```python
from build123d import *

# Parameters (mm, degrees)
ESQUISSE1_R        = 1.5
BOSS_EXTRU_1_DEPTH = 5


with BuildPart() as part:
    # Esquisse1 → Boss.-Extru.1 (new body)
    with BuildSketch(Plane(origin=(0, 0, 0), x_dir=(0, -1, 0), z_dir=(-1, 0, 0))):
        with BuildLine():
            Line((-5, 5), (-5, 0))
            Line((-5, 0), (0, 0))
            Line((0, 0), (0, 5))
            ThreePointArc((0, 5), (-2.5, 7.5), (-5, 5))
        make_face()
        with Locations(Location((-2.5, 5, 0), (0, 0, 270))):  # turned: the seam where the file's is
            Circle(ESQUISSE1_R, mode=Mode.SUBTRACT)
    extrude(amount=-BOSS_EXTRU_1_DEPTH)


solid = part.part
```
CAD build for the part. Positions are in the model's coordinates, mm. Coordinates: 2 decimals unless noted, no trailing zeros. Order: outer loops, then holes, each group sorted by start corner. A loop starts at its lowest first (then second) coordinate and runs counter-clockwise, first axis right, second up.
(1) Drill centre lines: L1, parallel to Y at x = 0.45, z = 5; L2, parallel to Z at x = 0.5, y = 3.6 (3 decimals); L3, parallel to Z at x = 4.3, y = 2.6. Where is each one in solid material? Low to high.
Solution:
L1: y = 0 to 1, 4 to 5
L2: z = 0 to 3.98, 6.02 to 7.245
L3: z = 0 to 3.5, 6.5 to 7.5
(2) Mould opens along Y. For faces 1 (the face through (2, 5, 3)), 2 (the face through (5, 3, 3)), 3 (the face through (2.5, 2.4, 7.5)), 4 (the face through (2.5, 3.4, 6.2)) say: released by +Y, released by -Y, zero draft, split by the parting line, or undercut.
Solution:
face 1: released by +Y
face 2: zero draft
face 3: split by the parting line
face 4: undercut
(3) Saw through at D-D, the plane y = 0.4. Write the cut outline in (x, z).
Solution:
outline: (0, 0) - (5, 0) - (5, 6.36) - (0, 6.36) - close
(4) Saw through at A-A, the plane y = 2.5. Write the cut outline in (x, z).
Solution:
outline: (0, 0) - (5, 0) - (5, 3.5) - (0, 3.5) - close; (0, 6.5) - (5, 6.5) - (5, 7.5) - (0, 7.5) - close
(5) Saw through at B-B, the plane x = 3.9. Write the cut outline in (y, z).
Solution:
outline: (0, 0) - (5, 0) - (5, 5) arc R2.5 ccw to (0, 5) - close; hole circle Ø3 at (2.5, 5)
(6) Saw through at C-C, the plane y = 1.6. Write the cut outline in (x, z).
Solution:
outline: (0, 0) - (5, 0) - (5, 3.8) - (0, 3.8) - close; (0, 6.2) - (5, 6.2) - (5, 7.33) - (0, 7.33) - close
